```python
from build123d import *

# Parameters (mm, degrees)
SKETCH1_W           = 400
SKETCH1_H           = 250
SKETCH1_W_2         = 15
SKETCH1_H_2         = 3.2
SKETCH1_W_3         = 3.2
SKETCH1_H_3         = 15
BOSS_EXTRUDE2_DEPTH = 3
FILLET1_R           = 10


with BuildPart() as part:
    # Sketch1 → Boss-Extrude2 (new body)
    with BuildSketch(Plane(origin=(0, 0, 0), x_dir=(1, 0, 0), z_dir=(0, 1, 0))):
        with Locations((200, 125)):
            Rectangle(SKETCH1_W, SKETCH1_H)
        with Locations((90, 4.6)):
            Rectangle(SKETCH1_W_2, SKETCH1_H_2, mode=Mode.SUBTRACT)
        with Locations((35, 4.6)):
            Rectangle(SKETCH1_W_2, SKETCH1_H_2, mode=Mode.SUBTRACT)
        with Locations((145, 4.6)):
            Rectangle(SKETCH1_W_2, SKETCH1_H_2, mode=Mode.SUBTRACT)
        with Locations((200, 4.6)):
            Rectangle(SKETCH1_W_2, SKETCH1_H_2, mode=Mode.SUBTRACT)
        with Locations((255, 4.6)):
            Rectangle(SKETCH1_W_2, SKETCH1_H_2, mode=Mode.SUBTRACT)
        with Locations((310, 4.6)):
            Rectangle(SKETCH1_W_2, SKETCH1_H_2, mode=Mode.SUBTRACT)
        with Locations((365, 4.6)):
            Rectangle(SKETCH1_W_2, SKETCH1_H_2, mode=Mode.SUBTRACT)
        with Locations((365, 245.4)):
            Rectangle(SKETCH1_W_2, SKETCH1_H_2, mode=Mode.SUBTRACT)
        with Locations((310, 245.4)):
            Rectangle(SKETCH1_W_2, SKETCH1_H_2, mode=Mode.SUBTRACT)
        with Locations((255, 245.4)):
            Rectangle(SKETCH1_W_2, SKETCH1_H_2, mode=Mode.SUBTRACT)
        with Locations((200, 245.4)):
            Rectangle(SKETCH1_W_2, SKETCH1_H_2, mode=Mode.SUBTRACT)
        with Locations((35, 245.4)):
            Rectangle(SKETCH1_W_2, SKETCH1_H_2, mode=Mode.SUBTRACT)
        with Locations((90, 245.4)):
            Rectangle(SKETCH1_W_2, SKETCH1_H_2, mode=Mode.SUBTRACT)
        with Locations((145, 245.4)):
            Rectangle(SKETCH1_W_2, SKETCH1_H_2, mode=Mode.SUBTRACT)
        with Locations((11.6, 95)):
            Rectangle(SKETCH1_W_3, SKETCH1_H_3, mode=Mode.SUBTRACT)
        with Locations((11.6, 35)):
            Rectangle(SKETCH1_W_3, SKETCH1_H_3, mode=Mode.SUBTRACT)
        with Locations((11.6, 155)):
            Rectangle(SKETCH1_W_3, SKETCH1_H_3, mode=Mode.SUBTRACT)
        with Locations((11.6, 215)):
            Rectangle(SKETCH1_W_3, SKETCH1_H_3, mode=Mode.SUBTRACT)
        with Locations((388.4, 35)):
            Rectangle(SKETCH1_W_3, SKETCH1_H_3, mode=Mode.SUBTRACT)
        with Locations((388.4, 95)):
            Rectangle(SKETCH1_W_3, SKETCH1_H_3, mode=Mode.SUBTRACT)
        with Locations((388.4, 155)):
            Rectangle(SKETCH1_W_3, SKETCH1_H_3, mode=Mode.SUBTRACT)
        with Locations((388.4, 215)):
            Rectangle(SKETCH1_W_3, SKETCH1_H_3, mode=Mode.SUBTRACT)
    extrude(amount=BOSS_EXTRUDE2_DEPTH)

    # Fillet1
    fillet1_edges = [part.edges().sort_by_distance(p)[0] for p in [
        (0, 1.5, -250),
        (400, 1.5, -250),
        (400, 1.5, 0),
        (0, 1.5, 0),
    ]]
    fillet(fillet1_edges, radius=FILLET1_R)


solid = part.part
```
Source: CAD feature listing. Evaluate the final solid. Frame: model axes, mm. Round coordinates to 2 decimals unless told otherwise and drop trailing zeros. Loops run counter-clockwise (first coordinate to the right, second up) from the corner with the lowest first, then second, coordinate; pieces in that order, holes last.
1. Section query A-A on z = -215. Output: boundary loops of the cut face in (x, y), and give its area (3 significant figures).
2. Section query B-B on x = 199. Output: boundary loops of the cut face in (y, z).
3. Contact query for a flat-ended pin moving along its axis: pin 1 (0.9 mm diameter, centred on y = 2, z = -245, fed in from +X). Output: stop coordinate, or through.
4. Ray query, L1, parallel to Z at x = 92, y = 1.1; L2, parallel to X at y = 0.25, z = -99. Return the intervals inside material, ascending.
Answers below:
1. outline: (0, 0) - (10, 0) - (10, 3) - (0, 3) - close; (13.2, 0) - (386.8, 0) - (386.8, 3) - (13.2, 3) - close; (390, 0) - (400, 0) - (400, 3) - (390, 3) - close
1. area: 1,180 mm2
2. outline: (0, -250) - (3, -250) - (3, -247) - (0, -247) - close; (0, -243.8) - (3, -243.8) - (3, -6.2) - (0, -6.2) - close; (0, -3) - (3, -3) - (3, 0) - (0, 0) - close
3. pin 1: stops at x = 398.9
4. L1: z = -250 to -247, -243.8 to -6.2, -3 to 0
4. L2: x = 0 to 10, 13.2 to 386.8, 390 to 400
